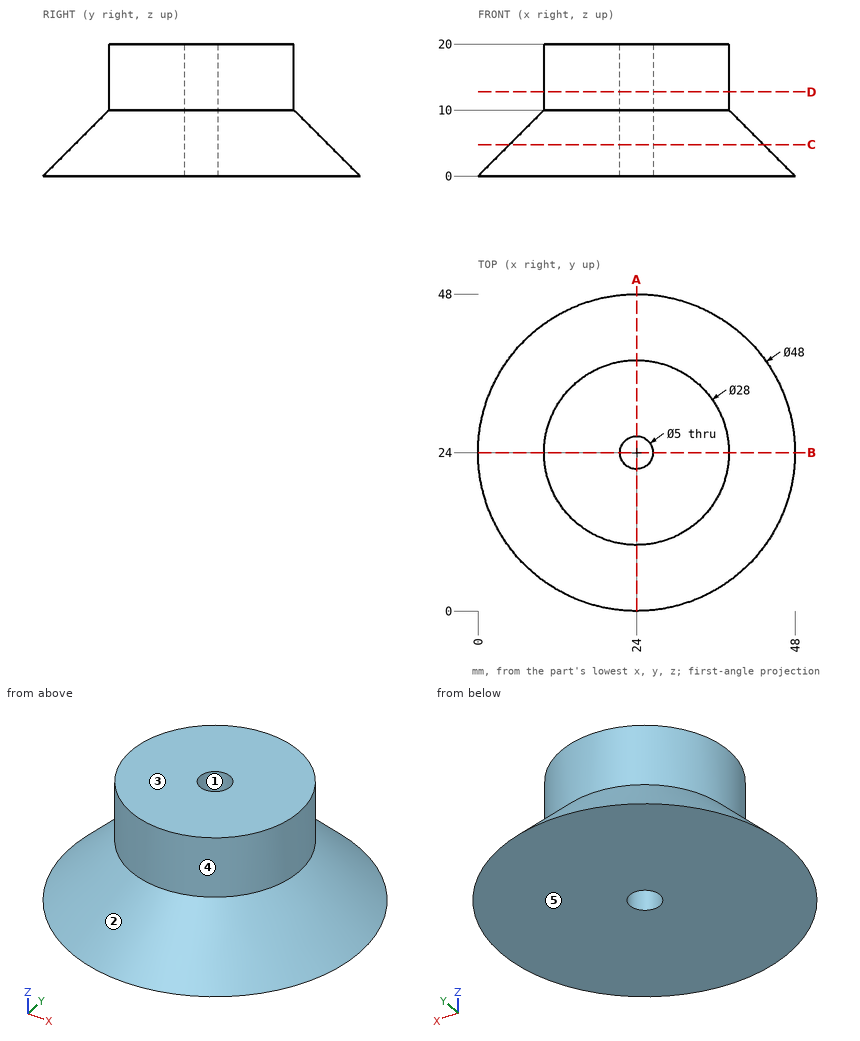
The drawing under review shows one solid part. Ordinate dimensions are in mm from its lowest x, y, z. A direction names the side the tool comes from. Coordinates: 2 decimals unless noted, no trailing zeros. Loops run counter-clockwise (first coordinate to the right, second up) from the corner with the lowest first, then second, coordinate; pieces in that order, holes last.
Item 1: Draft analysis for pull direction X (two halves, no side actions). For the marked faces 1, 2 and 3, state which applies: pulls with the +X half, pulls with the -X half, needs draft (parallel to the pull), parting line crosses it, or undercut.
Completed:
face 1: undercut
face 2: parting line crosses it
face 3: needs draft
Item 2: Add section C-C (z = 4.75). Write out the cut boundary in (x, y), and give its area (3 significant figures).
Completed:
outline: circle Ø38.5 at (24, 24); hole circle Ø5 at (24, 24)
area: 1,140 mm2
Item 3: Clearance check with flat-ended pins moving along their axes: pin 1 (5 mm diameter, centred on x = 13.5, y = 22, fed in from -Z); pin 2 (1.5 mm diameter, centred on x = 15, z = 10.5, fed in from +Y); pin 3 (10 mm diameter, centred on y = 35.5, z = 15, fed in from -X); pin 4 (1.5 mm diameter, centred on x = 11.5, y = 8, fed in from +Z). State where each tip first meets the part, or that it passes through.
Completed:
pin 1: stops at z = 0
pin 2: stops at y = 35.31
pin 3: stops at x = 11.6
pin 4: stops at z = 4.45
Item 4: Add section D-D (z = 12.75). Write out the cut boundary in (x, y).
Completed:
outline: circle Ø28 at (24, 24); hole circle Ø5 at (24, 24)
Item 5: Wall thickness on L1, parallel to Y at x = 24, z = 14.5; L2, parallel to Y at x = 26, z = 14.5: over which ranges is each line inside the solid? List them lowest first.
Completed:
L1: y = 10 to 21.5, 26.5 to 38
L2: y = 10.14 to 22.5, 25.5 to 37.86
Item 6: For the marked faces 4 and 5, list the 3-axis set-ups (+Z, -Z, +X, -X, +Y, -Y) from which the entire face can be reached by the end or side of a thin tool; tool diameter is ignored.
Completed:
face 4: +Z
face 5: -Z, +X, -X, +Y, -Y
Item 7: Add section A-A (x = 24). Write out the cut boundary in (y, z), and give its area (3 significant figures).
Completed:
outline: (0, 0) - (21.5, 0) - (21.5, 20) - (10, 20) - (10, 10) - close; (26.5, 0) - (48, 0) - (38, 10) - (38, 20) - (26.5, 20) - close
area: 560 mm2
